Autodesk Fusion 360 part; units mm, degrees
sketch "Skizze1" plane through (0, 0, 0) normal (0, 1, 0) x (1, 0, 0)
  line L0 (0, 0) -> (-39.3, 0)
  line L1 (-39.3, 0) -> (-39.3, -128.5)
  line L2 (-39.3, -128.5) -> (0, -128.5)
  line L3 (0, -128.5) -> (0, 0)
  line L4 (0, 0) -> (-7, 0)
  line L5 (-7, 0) -> (-7, -3)
  line L6 (-39.3, -128.5) -> (-32.3, -128.5)
  line L7 (-32.3, -128.5) -> (-32.3, -125.5)
  line L8 (-7, -3) -> (-9, -3)
  line L9 (-7, -3) -> (-5, -3)
  circle A0 centre (-5, -3) radius 1.5
  circle A1 centre (-9, -3) radius 1.5
  line L10 (-9, -3) -> (-9, -1.5)
  line L11 (-9, -1.5) -> (-5, -1.5)
  line L12 (-9, -4.5) -> (-5, -4.5)
  line L13 (-32.3, -125.5) -> (-34.3, -125.5)
  line L14 (-32.3, -125.5) -> (-30.3, -125.5)
  circle A2 centre (-34.3, -125.5) radius 1.5
  circle A3 centre (-30.3, -125.5) radius 1.5
  line L15 (-34.3, -125.5) -> (-34.3, -124)
  line L16 (-30.3, -125.5) -> (-30.3, -124)
  line L17 (-34.3, -124) -> (-30.3, -124)
  line L18 (-34.3, -125.5) -> (-34.3, -127)
  line L19 (-34.3, -127) -> (-30.3, -127)
  line L20 (0, -128.5) -> (-10, -128.5)
  line L21 (-10, -128.5) -> (-10, -16.5842)
  circle A4 centre (-10, -97.2748) radius 3.5
  line L22 (-10, -97.2748) -> (-10, -76.7748)
  circle A5 centre (-10, -76.7748) radius 3.5
  line L23 (-10, -76.7748) -> (-21.5, -76.7748)
  line L24 (-21.5, -76.7748) -> (-21.5, -39.6569)
  line L25 (-21.5, -76.7748) -> (-21.5, -50.7748)
  line L26 (-21.5, -50.7748) -> (-17.1, -50.7748)
  circle A6 centre (-17.1, -50.7748) radius 3.25
  line L27 (-39.3, 0) -> (-39.3, -25)
  line L28 (-39.3, -25) -> (0, -25)
  line L29 (0, -25) -> (-19.65, -25)
  circle A7 centre (-9.825, -25) radius 3.25
  line L30 (-19.65, -25) -> (-39.3, -25)
  circle A8 centre (-29.475, -25) radius 3.25
  dimension "d1" = 39.3
  dimension "d2" = 128.5
  dimension "d3" = 7
  dimension "d4" = 3
  dimension "d5" = 7
  dimension "d6" = 3
  dimension "d7" = 2
  dimension "d8" = 2
  dimension "d9" = 3
  dimension "d10" = 3
  dimension "d11" = 2
  dimension "d12" = 2
  dimension "d13" = 3
  dimension "d14" = 3
  dimension "d15" = 10
  dimension "d16" = 7
  dimension "d17" = 20.5
  dimension "d18" = 7
  dimension "d19" = 11.5
  dimension "d20" = 26
  dimension "d21" = 4.4
  dimension "d22" = 6.5
  dimension "d23" = 25
  dimension "d24" = 6.5
  dimension "d25" = 6.5
extrude "Extrusion1" add sketch "Skizze1" along normal blind 2 contours L0 L1 L3 L4 L27 L28 L29 A7 L30 A8 | L2 L3 L20 L21 A4 L22 A5 L28 L29 A7 | L1 L2 L6 L21 A4 L22 A5 L28 L29 A7 L30 A8
sketch "Skizze2" plane through (0, 2, 0) normal (0, 1, 0) x (-1, 0, 0)
  circle A0 centre (9.825, 25) radius 3.25
  arc A1 (9, 1.5) -> (9, 4.5) centre (9, 3) ccw
  line L0 (9, 1.5) -> (5, 1.5)
  arc A2 (5, 4.5) -> (5, 1.5) centre (5, 3) ccw
  line L1 (5, 4.5) -> (9, 4.5)
  arc A3 (34.3, 124) -> (34.3, 127) centre (34.3, 125.5) ccw
  line L2 (34.3, 124) -> (30.3, 124)
  arc A4 (30.3, 127) -> (30.3, 124) centre (30.3, 125.5) ccw
  line L3 (30.3, 127) -> (34.3, 127)
  circle A5 centre (10, 76.7748) radius 3.5
  circle A6 centre (10, 97.2748) radius 3.5
  circle A7 centre (17.1, 50.7748) radius 3.25
  circle A8 centre (29.475, 25) radius 3.25
  line L4 (0, 128.5) -> (0, 0)
  line L5 (0, 0) -> (39.3, 0)
  line L6 (39.3, 0) -> (39.3, 128.5)
  line L7 (39.3, 128.5) -> (0, 128.5)
extrude "Extrusion2" add sketch "Skizze2" against normal blind 2 contours A0 | A5 | A6 | A7 | A8
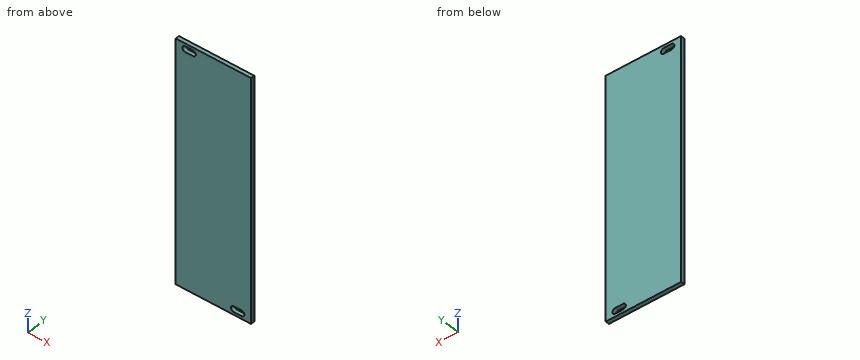
The listing builds one solid part. Answer for the finished solid, in the listing's coordinates (mm). Give positions to 0.01 mm unless a question says otherwise; leave off trailing zeros. Loops run counter-clockwise (first coordinate to the right, second up) from the corner with the lowest first, then second, coordinate; pieces in that order, holes last. Notation, with made-up numbers: (14, 51) - (29, 51) arc R18 ccw to (29, 77) - close; hole circle Ø10 at (19, 60.25). An arc over 180 degrees is marked (long way). Answer as a JSON object with one key per item and string values.
1. A cutting plane is placed at A-A (z = 125.5). Write down the section's boundary in (x, y), then the cut area to 3 significant figures.
Determined:
{"outline": "(-39.3, 0) - (-35.8, 0) - (-35.8, 2) - (-39.3, 2) - close; (-28.8, 0) - (0, 0) - (0, 2) - (-28.8, 2) - close", "area": "64.6 mm²"}
2. Find the intervals of material crossed by L1, parallel to Z at x = -33, y = 0.9; L2, parallel to Z at x = -9, y = 1.6, in increasing order. Write a range as [from, to].
Determined:
{"L1": "[0, 124], [127, 128.5]", "L2": "[0, 1.5], [4.5, 128.5]"}
3. A flat-ended cylindrical pin translates along its axis: pin 1 Ø0.6 at (x, y) = (-32.5, 1) entering from -Z. Find the tip coordinate at first contact, or state that the pin passes through.
Determined:
{"pin 1": "z = 0"}
